from build123d import *

# Parameters (mm, degrees)
EXTRUDE_1_DEPTH                  = 75
CUT_EXTRUDE_1_DEPTH              = 69
SKETCH_4_W                       = 160
SKETCH_4_H                       = 69
CUT_EXTRUDE_2_DEPTH              = 157
SKETCH_5_R                       = 2.5
CUT_EXTRUDE_3_DEPTH              = 348.108052341
CUT_EXTRUDE_16_REACH             = 349.108
SKETCH_6_R                       = 2.5
CUT_EXTRUDE_18_REACH             = 349.743
SKETCH_8_R                       = 5
CUT_EXTRUDE_19_REACH             = 349.743
SKETCH_9_R                       = 5
CUT_EXTRUDE_20_DEPTH             = 348.742720988
CUT_EXTRUDE_20_DEPTH_BACK        = 348.742720988
SKETCH_10_R                      = 2.5
CUT_EXTRUDE_21_REACH             = 349.743
SKETCH_11_R                      = 5
CUT_EXTRUDE_21_DIRECTION_2_DEPTH = 348.742720988
EXTRUDE_2_DEPTH                  = 69


with BuildPart() as part:
    # 草图1 → 凸台-拉伸1 (new body)
    with BuildSketch(Plane(origin=(0, 0, 0), x_dir=(1, 0, 0), z_dir=(0, 1, 0))):
        with BuildLine():
            Line((0, 80), (250, 80))
            ThreePointArc((250, 80), (330, 0), (250, -80))
            Line((250, -80), (0, -80))
            ThreePointArc((0, -80), (-80, 0), (0, 80))
        make_face()
    extrude(amount=EXTRUDE_1_DEPTH)

    # 草图3 → 切除-拉伸1 (cut)
    with BuildSketch(Plane(origin=(0, 72, 0), x_dir=(1, 0, 0), z_dir=(0, 1, 0))):
        with BuildLine():
            Line((0, 77), (250, 77))
            ThreePointArc((250, 77), (327, 0), (250, -77))
            Line((250, -77), (0, -77))
            ThreePointArc((0, -77), (-77, 0), (0, 77))
        make_face()
    extrude(amount=-CUT_EXTRUDE_1_DEPTH, mode=Mode.SUBTRACT)

    # 草图4 → 切除-拉伸2 (cut)
    with BuildSketch(Plane(origin=(0, 0, -80), x_dir=(-1, 0, 0), z_dir=(0, 0, -1))):
        with Locations((0, 37.5)):
            Rectangle(SKETCH_4_W, SKETCH_4_H)
        with Locations((-250, 37.5)):
            Rectangle(SKETCH_4_W, SKETCH_4_H)
    extrude(amount=-CUT_EXTRUDE_2_DEPTH, mode=Mode.SUBTRACT)

    # 草图5 → 切除-拉伸3 (cut, through all)
    with BuildSketch(Plane(origin=(0, 3, 0), x_dir=(1, 0, 0), z_dir=(0, 1, 0))):
        with Locations(Location((0, 0, 0), (0, 0, 270))):
            Circle(SKETCH_5_R)
    extrude(amount=-CUT_EXTRUDE_3_DEPTH, mode=Mode.SUBTRACT)

    # 草图6 → 切除-拉伸16 (cut, up to next)
    with BuildSketch(Plane(origin=(0, 72, 0), x_dir=(1, 0, 0), z_dir=(0, 1, 0)), mode=Mode.PRIVATE) as cut_extrude_16_sk1:
        with Locations(Location((0, 0, 0), (0, 0, 270))):
            Circle(SKETCH_6_R)
    cut_extrude_16_tool1 = extrude(cut_extrude_16_sk1.sketch, amount=CUT_EXTRUDE_16_REACH, mode=Mode.PRIVATE) & part.part
    add(cut_extrude_16_tool1.solids().sort_by_distance((0, 72, 0))[0], mode=Mode.SUBTRACT)

    # 草图8 → 切除-拉伸18 (cut, up to next)
    with BuildSketch(Plane(origin=(0, 0, 0), x_dir=(-1, 0, 0), z_dir=(0, -1, 0)), mode=Mode.PRIVATE) as cut_extrude_18_sk1:
        with Locations(Location((0, -61.25, 0), (0, 0, 90))):
            Circle(SKETCH_8_R)
    cut_extrude_18_tool1 = extrude(cut_extrude_18_sk1.sketch, amount=-CUT_EXTRUDE_18_REACH, mode=Mode.PRIVATE) & part.part
    add(cut_extrude_18_tool1.solids().sort_by_distance((0, 0, 61.25))[0], mode=Mode.SUBTRACT)

    # 草图9 → 切除-拉伸19 (cut, up to next)
    with BuildSketch(Plane.XZ, mode=Mode.PRIVATE) as cut_extrude_19_sk1:
        with Locations(Location((0, -61.25, 0), (0, 0, 270))):
            Circle(SKETCH_9_R)
    cut_extrude_19_tool1 = extrude(cut_extrude_19_sk1.sketch, amount=-CUT_EXTRUDE_19_REACH, mode=Mode.PRIVATE) & part.part
    add(cut_extrude_19_tool1.solids().sort_by_distance((0, 0, -61.25))[0], mode=Mode.SUBTRACT)

    # 草图10 → 切除-拉伸20 (cut, two sides: drawn at the far end of the back side and taken through both)
    with BuildSketch(Plane(origin=(0, 75, 0), x_dir=(1, 0, 0), z_dir=(0, 1, 0)).offset(-CUT_EXTRUDE_20_DEPTH_BACK)):
        with Locations(Location((250, 0, 0), (0, 0, 270))):
            Circle(SKETCH_10_R)
    extrude(amount=CUT_EXTRUDE_20_DEPTH + CUT_EXTRUDE_20_DEPTH_BACK, mode=Mode.SUBTRACT)

    # 草图11 → 切除-拉伸21 (cut, up to next)
    with BuildSketch(Plane.XZ, mode=Mode.PRIVATE) as cut_extrude_21_sk1:
        with Locations(Location((250, 61.25, 0), (0, 0, 90))):
            Circle(SKETCH_11_R)
    cut_extrude_21_tool1 = extrude(cut_extrude_21_sk1.sketch, amount=-CUT_EXTRUDE_21_REACH, mode=Mode.PRIVATE) & part.part
    # 草图11 → 切除-拉伸21 (cut, up to next)
    with BuildSketch(Plane.XZ, mode=Mode.PRIVATE) as cut_extrude_21_sk2:
        with Locations(Location((250.041254048, -61.25, 0), (0, 0, 90))):
            Circle(SKETCH_11_R)
    cut_extrude_21_tool2 = extrude(cut_extrude_21_sk2.sketch, amount=-CUT_EXTRUDE_21_REACH, mode=Mode.PRIVATE) & part.part
    add(cut_extrude_21_tool1.solids().sort_by_distance((250, 0, 61.25))[0], mode=Mode.SUBTRACT)
    add(cut_extrude_21_tool2.solids().sort_by_distance((250.041254, 0, -61.25))[0], mode=Mode.SUBTRACT)

    # 草图11 → 切除-拉伸21 direction 2 (cut)
    with BuildSketch(Plane.XZ):
        with Locations(Location((250, 61.25, 0), (0, 0, 90))):
            Circle(SKETCH_11_R)
        with Locations(Location((250.041254048, -61.25, 0), (0, 0, 90))):
            Circle(SKETCH_11_R)
    extrude(amount=CUT_EXTRUDE_21_DIRECTION_2_DEPTH, mode=Mode.SUBTRACT)

    # 草图12 → 凸台-拉伸2 (add)
    with BuildSketch(Plane(origin=(0, 72, 0), x_dir=(1, 0, 0), z_dir=(0, 1, 0))):
        Polygon((84.732642754, 80), (116.111672897, -2.332361516), (88.187612247, -80), (102.698484118, -80), (123.448818124, -21.583577713), (145.712854307, -80), (156.94150516, -80), (128.865571981, -6.33431085), (159.53273228, 80), (145.712854307, 80), (121.562315366, 12.827988338), (95.961293606, 80), align=None)
    extrude(amount=-EXTRUDE_2_DEPTH)


solid = part.part
CAD build for the part. Positions are in the model's coordinates, mm. A direction names the side the tool comes from. Round coordinates to 2 decimals unless told otherwise and drop trailing zeros. Write each loop counter-clockwise with the first axis right and the second up, starting at its lowest first coordinate (ties: lowest second). Pieces come first, ordered by that corner, then holes. Notation, with made-up numbers: M -25,57.5 L -7,57.5 A33 cw -7,91.5 Z; hole C -17,60 d4. An arc over 180 degrees is marked long. Put each result on its own line as item: value. Start each with the question number.
1) Saw through at A-A, the plane x = 287.5. Write the cut outline in (y, z).
2) Pull direction Y, two halves, no side cores. Call faces 4 (the flat face through (126, 40, -80)), 5 (the flat face through (215, 38, 77)): pulls with the +Y half, pulls with the -Y half, needs draft (parallel to the pull), parting line crosses it, or undercut.
3) 3-axis set-ups, long thin cutter, end or side, ignore diameter. For faces 1 (the flat face through (121, 72, -52)), 2 (the flat face through (231, 72, -3)), 3 (the cylindrical face through (245.043, 1.479, 60.599)): which of +Z, -Z, +X, -X, +Y, -Y reach the whole face in a straight line?
4) Saw through at B-B, the plane y = 44. Write the cut outline in (x, z), and give its area (3 significant figures).
5) Pin check, flat tips, straight feed: pin 1 Ø2 at (y, z) = (64, 61.5) entering from -X; pin 2 Ø4 at (y, z) = (59, -28.5) entering from +X; pin 3 Ø1.5 at (y, z) = (28.5, -78) entering from +X. Stop position of each tip, or through.
6) Saw through at D-D, the plane x = 239. Write the cut outline in (y, z), and give its area (3 significant figures).
7) Drill centre lines: probe 1 along Z at (x, y) = (250, 0.6); probe 2 along X at (y, z) = (73, 0); probe 3 along Y at (x, z) = (-43.5, 0). Where is each one in solid material? Low to high. Write a range as [from, to].
8) Saw through at C-C, the plane z = -34.5. Write the cut outline in (x, y).
Resolved:
1. outline: M 0,-70.67 L 3,-70.67 L 3,70.67 L 0,70.67 Z; M 72,-70.67 L 75,-70.67 L 75,70.67 L 72,70.67 Z
2. face 4: needs draft
2. face 5: undercut
3. face 1: none
3. face 2: +X
3. face 3: -Y
4. outline: M -21.7,77 L 89.27,77 L 116.11,2.33 L 85.88,-77 L 80,-77 L 80,-80 L 170,-80 L 170,-77 L 158.47,-77 L 128.87,6.33 L 155.8,77 L 271.7,77 A80 ccw 250,80 L 0,80 A80 ccw Z; hole M 97.1,-77 L 144.63,-77 L 121.56,-12.83 Z; hole M 103.76,77 L 123.45,21.58 L 144.57,77 Z
4. area: 4,800 mm²
5. pin 1: x = 94.48
5. pin 2: x = 141.95
5. pin 3: x = 170
6. outline: M 0,-80 L 3,-80 L 3,77 L 72,77 L 72,-80 L 75,-80 L 75,80 L 0,80 Z
6. area: 1,170 mm²
7. probe 1: [-80, -66.25], [-56.25, -2.5], [2.5, 56.25], [66.25, 80]
7. probe 2: [-80, -2.5], [2.5, 247.5], [252.5, 330]
7. probe 3: [0, 3], [72, 75]
8. outline: M -72.18,0 L 322.18,0 L 322.18,3 L 143.37,3 L 143.37,72 L 322.18,72 L 322.18,75 L -72.18,75 L -72.18,72 L 102.07,72 L 102.07,3 L -72.18,3 Z; hole M 113.3,3 L 129.35,3 L 129.35,72 L 113.3,72 Z
